from build123d import *

# Parameters (mm, degrees)
SIDES_W              = 11.8
SIDES_H              = 10.45
SIDES_W_2            = 9
SIDES_H_2            = 10.7
SIDES_EXTRUDED_DEPTH = 3


with BuildPart() as part:
    # Sides → Sides Extruded (new body)
    with BuildSketch(Plane(origin=(0, 0, 0), x_dir=(0, 0, -1), z_dir=(1, 0, 0))):
        Polygon((0, 16.66666666), (0, 25), (20, 25), (20, 28), (40, 28), (40, 25), (60, 25), (60, 16.66666666), (57, 16.66666666), (57, 8.33333333), (60, 8.33333333), (60, 0), (40, 0), (40, -3), (20, -3), (20, 0), (0, 0), (0, 8.33333333), (3, 8.33333333), (3, 16.66666666), align=None)
        with Locations((44.6, 10.225)):
            Rectangle(SIDES_W, SIDES_H, mode=Mode.SUBTRACT)
        with Locations((14.2, 9.35)):
            Rectangle(SIDES_W_2, SIDES_H_2, mode=Mode.SUBTRACT)
    extrude(amount=SIDES_EXTRUDED_DEPTH)


solid = part.part
Input: part model. Units: mm. Frame: model coordinates. A direction names the side the tool comes from. Give positions to 0.01 mm unless a question says otherwise; leave off trailing zeros. Write each loop counter-clockwise with the first axis right and the second up, starting at its lowest first coordinate (ties: lowest second). Pieces come first, ordered by that corner, then holes. Notation, with made-up numbers: M 74.25,66 L 131.25,66 A23 ccw 131.25,84 Z; hole C 40,15 d8. An arc over 180 degrees is marked long. Write item = value, one per line. Start each with the question number.
1) Reachability of faces 1 (the flat face through (1, 10, -50.5)), 2 (the flat face through (1, 13, -57)), 3 (the flat face through (1, 25, -10)) from +Z, -Z, +X, -X, +Y, -Y: full face, straight path, thin tool, end or side. Return the list, or none.
2) Material intervals for line 1 along Z through (x, y) = (0.35, 5.5); line 2 along Z through (x, y) = (1.8, 14); line 3 along Y through (x, z) = (1.3, -48.5), sorted ascending. Write a range as [from, to].
3) Draft query along Y for faces 4 (the flat face through (1, 16.667, -59)), 5 (the flat face through (1, 0, -50)), 6 (the flat face through (1, 4, -60)). Return one class per face: +Y half, -Y half, draft (parallel to the pull), parting line (faces both ways), or undercut.
4) Cut plane C-C on z = -44.5. Return the cut outline in (x, y), then the cut area to 4 significant figures.
5) Cut plane A-A on z = -11. Return the cut outline in (x, y).
6) First-contact query: pin 1 Ø1.5 at (x, z) = (2, -58) entering from -Y; pin 2 Ø0.9 at (x, y) = (1.5, 12.5) entering from +Z; pin 3 Ø1.5 at (x, y) = (1.5, 13) entering from -Z. Flat tips, straight axial feed; report the tip coordinate or a pass-through.
7) Cut plane B-B on x = 0.45. Return the cut outline in (y, z).
Solved:
q1.face_1 = +X, -X
q1.face_2 = -Z, +X, -X
q1.face_3 = +Z, +X, -X, +Y
q2.line_1 = [-60, -50.5], [-38.7, -18.7], [-9.7, 0]
q2.line_2 = [-57, -50.5], [-38.7, -18.7], [-9.7, -3]
q2.line_3 = [0, 5], [15.45, 25]
q3.face_4 = undercut
q3.face_5 = -Y half
q3.face_6 = draft
q4.outline = M 0,0 L 3,0 L 3,5 L 0,5 Z; M 0,15.45 L 3,15.45 L 3,25 L 0,25 Z
q4.area = 43.65 mm2
q5.outline = M 0,0 L 3,0 L 3,4 L 0,4 Z; M 0,14.7 L 3,14.7 L 3,25 L 0,25 Z
q6.pin_1 = 0
q6.pin_2 = -3
q6.pin_3 = -57
q7.outline = M -3,-40 L 0,-40 L 0,-60 L 8.33,-60 L 8.33,-57 L 16.67,-57 L 16.67,-60 L 25,-60 L 25,-40 L 28,-40 L 28,-20 L 25,-20 L 25,0 L 16.67,0 L 16.67,-3 L 8.33,-3 L 8.33,0 L 0,0 L 0,-20 L -3,-20 Z; hole M 4,-18.7 L 14.7,-18.7 L 14.7,-9.7 L 4,-9.7 Z; hole M 5,-50.5 L 15.45,-50.5 L 15.45,-38.7 L 5,-38.7 Z
